```python
from build123d import *


with BuildPart() as f1:
    # F0 (on Front) → F1 (revolve)
    with BuildSketch(Plane.XZ):
        Polygon((64.421296, -7.356068), (41.684367, -7.356068), (41.684367, -45.696769), (41.684367, -49.709167), (41.684367, -58.179785), (64.421296, -58.179785), (64.421296, -49.709167), align=None)
        Polygon((63.083835, 51.938269), (63.083835, 17.164147), (92.062272, 17.164147), (92.953913, 43.467648), (92.953913, 51.938269), align=None)
        Polygon((92.953913, 43.467648), (92.062272, 17.164147), (106.328569, 17.164147), (115.358189, 6.462383), (123.450934, 6.462383), (124.607272, 36.334496), (124.607272, 43.467648), align=None)
        Polygon((123.450934, 6.462383), (115.358189, 6.462383), (106.328569, -7.356068), (89.833163, -7.356068), (89.833163, -40.346902), (121.932343, -40.346902), (121.932343, -32.767929), align=None)
        Polygon((183.009967, 6.462383), (123.450934, 6.462383), (121.932343, -32.767929), (168.74367, -32.767929), (183.009967, -20.730732), align=None)
        Polygon((89.833163, -7.356068), (64.421296, -7.356068), (64.421296, -49.709167), (89.833163, -49.709167), (89.833163, -40.346902), align=None)
        Polygon((40.792722, 17.164147), (0, 17.164147), (0, 8.693527), (92.062272, 8.693527), (99.641241, 5.12695), (91.170624, 0), (0, 0), (0, -7.356068), (41.684367, -7.356068), (64.421296, -7.356068), (89.833163, -7.356068), (106.328569, -7.356068), (115.358189, 6.462383), (106.328569, 17.164147), (92.062272, 17.164147), (63.083835, 17.164147), align=None)
        Polygon((40.792722, 51.938269), (40.792722, 17.164147), (63.083835, 17.164147), (63.083835, 51.938269), (63.083835, 59.071422), (40.792722, 59.071422), align=None)
        Polygon((124.607272, 36.334496), (123.450934, 6.462383), (183.009967, 6.462383), (183.009967, 23.851477), (166.960374, 36.334496), align=None)
        Polygon((92.062272, 8.693527), (0, 8.693527), (0, 0), (91.170624, 0), (99.641241, 5.12695), align=None)
        Polygon((41.684367, -7.356068), (0, -7.356068), (0, -39.901081), (15.826687, -49.709167), (41.684367, -49.709167), (41.684367, -45.696769), align=None)
        Polygon((15.826687, 51.938269), (0, 39.901074), (0, 17.164147), (40.792722, 17.164147), (40.792722, 51.938269), align=None)
    revolve(axis=Axis((0, 0, -4e-06), (0, 0, -1)))


solid = f1.part
```
Source: CAD feature listing. Evaluate the final solid. Frame: model axes, mm. A direction names the side the tool comes from. Coordinates: 2 decimals unless noted, no trailing zeros. Write each loop counter-clockwise with the first axis right and the second up, starting at its lowest first coordinate (ties: lowest second). Pieces come first, ordered by that corner, then holes. Notation, with made-up numbers: M 80.5,-2.75 L 93.5,-2.75 A24 cw 93.5,36.25 Z; hole C -6.75,75.25 d3. An arc over 180 degrees is marked long. Answer as a JSON object with one key per item and string values.
1. Draft query along X for faces 1 (the flat face through (-93, 9, 43.468)), 2 (the cylindrical face through (60.17, -18.95, 55.55)), 3 (the flat face through (-18, -1, -49.709)). Return one class per face: released by +X, released by -X, zero draft, split by the parting line, or undercut.
Evaluation:
{"face 1": "zero draft", "face 2": "split by the parting line", "face 3": "undercut"}
2. Contact query for flat-ended pins moving along their axis: P1, Ø8, axis at x = 48.5, z = -1, coming from the -Y side; P2, Ø3, axis at x = 44, z = 9.5, coming from the +Y side; P3, Ø2, axis at x = -115, y = 28.5, coming from the -Z side. Output: stop coordinate, or through.
Evaluation:
{"P1": "y = -177.52", "P2": "y = 178.01", "P3": "z = -40.35"}
3. Cut plane A-A on z = -9. Output: boundary loops of the cut face in (x, y).
Evaluation:
{"outline": "C 0,0 d366.02"}
4. Ray query, L1, parallel to X at y = 0, z = 55.25; L2, parallel to Y at x = 0, z = -56.25. Return the intervals inside material, ascending.
Evaluation:
{"L1": "-63.08 to -40.79, 40.79 to 63.08", "L2": "-64.42 to -41.68, 41.68 to 64.42"}
5. Access query for faces 4 (the flat face through (10, 90, -40.347)), 5 (the flat face through (-1, 41, 59.071)), 6 (the cylindrical face through (49.97, -78.38, 47.76)). Directions: +Z, -Z, +X, -X, +Y, -Y. A direction counts if a zero-diameter tool reaches every point of the face in a straight line with its end or side. Return the directions, or none.
Evaluation:
{"face 4": "-Z", "face 5": "+Z, +X, -X, +Y, -Y", "face 6": "+Z"}
